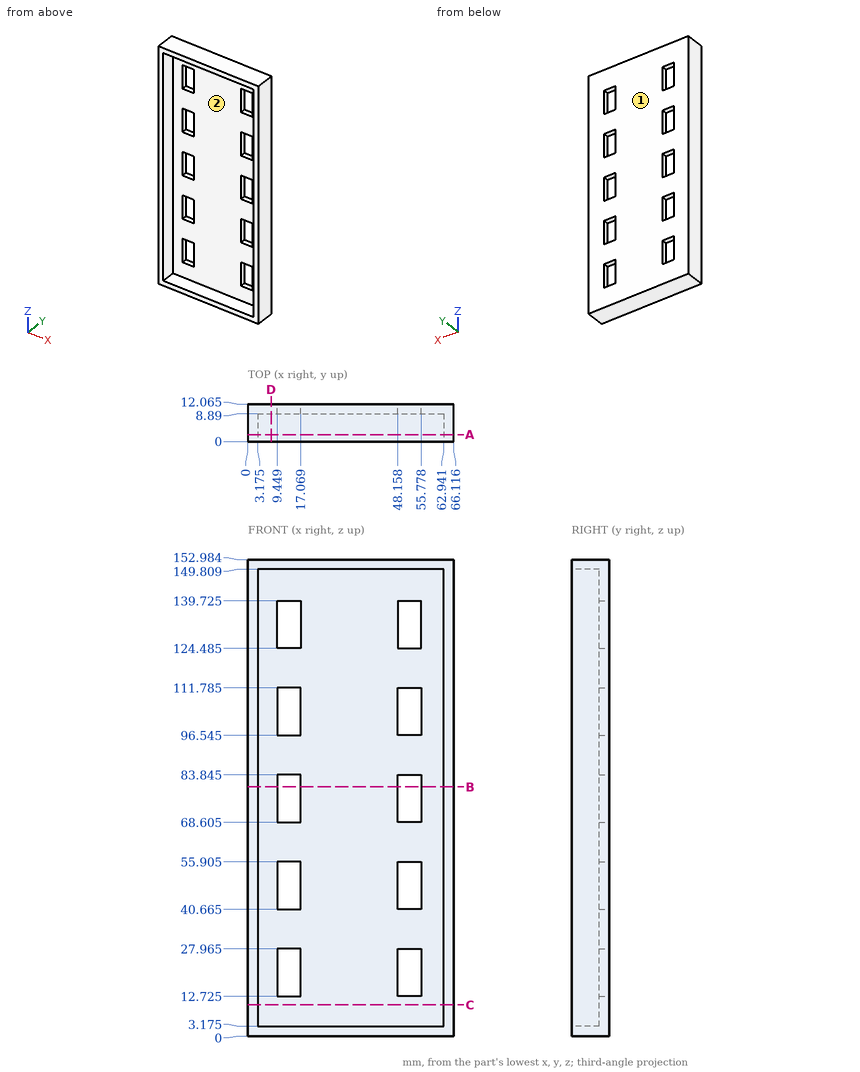
Geometry: see drawing. Coordinates: mm, zero at the bounding-box minimum. Coordinates: 2 decimals unless noted, no trailing zeros. Write each loop counter-clockwise with the first axis right and the second up, starting at its lowest first coordinate (ties: lowest second). Pieces come first, ordered by that corner, then holes. Notation, with made-up numbers: (71.5, 35) - (105.5, 35) arc R13 ccw to (105.5, 39) - close; hole circle Ø10 at (-1.75, 20.5). An arc over 180 degrees is marked (long way). Put each result on its own line as item: value. Start each with the question number.
1) Cut plane B-B (z = 80). Return the cut outline in (x, y) (1 decimal), plus the area to 3 significant figures.
2) Cut plane C-C (z = 10). Return the cut outline in (x, y) (1 decimal).
3) Cut plane A-A (y = 2.25). Return the cut outline in (x, z) (1 decimal).
4) Contact query for flat-ended pins moving along their axis: pin 1 (1 mm diameter, centred on x = 13.5, y = 11, fed in from -Z); pin 2 (1 mm diameter, centred on x = 48, z = 135, fed in from -Y). Output: stop coordinate, or through.
5) Cut plane D-D (x = 7.5). Return the cut outline in (y, z) (1 decimal), plus the area to 3 significant figures.
6) Mould query, pull axis Z, two halves, no side actions, for the marked faces 1 and 2. Classes: pulls with the +Z half, pulls with the -Z half, needs draft (parallel to the pull), parting line crosses it, or undercut.
7) Ray query, L1, parallel to Z at x = 50.5, y = 10.75 (1 decimal); L2, parallel to X at y = 11, z = 128.5; L3, parallel to Z at x = 57, y = 7 (1 decimal). Return the intervals inside material, ascending.
Resolved:
1. outline: (0, 0) - (3.2, 0) - (3.2, 8.9) - (9.4, 8.9) - (9.4, 12.1) - (0, 12.1) - close; (17.1, 8.9) - (48.2, 8.9) - (48.2, 12.1) - (17.1, 12.1) - close; (55.8, 8.9) - (62.9, 8.9) - (62.9, 0) - (66.1, 0) - (66.1, 12.1) - (55.8, 12.1) - close
1. area: 218 mm2
2. outline: (0, 0) - (3.2, 0) - (3.2, 8.9) - (62.9, 8.9) - (62.9, 0) - (66.1, 0) - (66.1, 12.1) - (0, 12.1) - close
3. outline: (0, 0) - (66.1, 0) - (66.1, 153) - (0, 153) - close; hole (3.2, 3.2) - (62.9, 3.2) - (62.9, 149.8) - (3.2, 149.8) - close
4. pin 1: stops at z = 0
4. pin 2: stops at y = 8.89
5. outline: (0, 0) - (12.1, 0) - (12.1, 153) - (0, 153) - (0, 149.8) - (8.9, 149.8) - (8.9, 3.2) - (0, 3.2) - close
5. area: 542 mm2
6. face 1: needs draft
6. face 2: undercut
7. L1: z = 0 to 12.7, 28 to 40.7, 55.9 to 68.6, 83.8 to 96.5, 111.8 to 124.5, 139.7 to 153
7. L2: x = 0 to 9.45, 17.07 to 48.16, 55.78 to 66.12
7. L3: z = 0 to 3.2, 149.8 to 153
